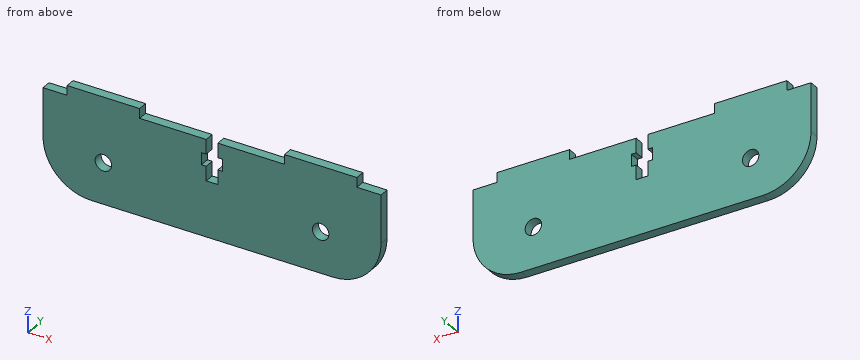
```python
from build123d import *

# Parameters (mm, degrees)
SKETCH_1_W          = 70
SKETCH_1_H          = 20
SKETCH_1_R          = 1.7
EXTRUDE_1_DEPTH     = 2
CUT_EXTRUDE_1_DEPTH = 2
SKETCH_3_W          = 15
SKETCH_3_H          = 2
EXTRUDE_2_DEPTH     = 2
FILLET_1_R          = 10


with BuildPart() as part:
    # 草图1 → 凸台-拉伸1 (new body)
    with BuildSketch(Plane(origin=(0, 0, 0), x_dir=(1, 0, 0), z_dir=(0, 1, 0))):
        with Locations((35, -10)):
            Rectangle(SKETCH_1_W, SKETCH_1_H)
        with Locations(Location((57.5, -8.5, 0), (0, 0, 270))):
            Circle(SKETCH_1_R, mode=Mode.SUBTRACT)
        with Locations(Location((12.5, -8.5, 0), (0, 0, 270))):
            Circle(SKETCH_1_R, mode=Mode.SUBTRACT)
    extrude(amount=EXTRUDE_1_DEPTH)

    # 草图2 → 切除-拉伸1 (cut)
    with BuildSketch(Plane(origin=(0, 2, 0), x_dir=(1, 0, 0), z_dir=(0, 1, 0))):
        Polygon((33.8, -20), (33.8, -17), (32.8, -17), (32.8, -14.5), (33.8, -14.5), (33.8, -11.5), (36.2, -11.5), (36.2, -14.5), (37.2, -14.5), (37.2, -17), (36.2, -17), (36.2, -20), align=None)
    extrude(amount=-CUT_EXTRUDE_1_DEPTH, mode=Mode.SUBTRACT)

    # 草图3 → 凸台-拉伸2 (add)
    with BuildSketch(Plane(origin=(0, 2, 0), x_dir=(1, 0, 0), z_dir=(0, 1, 0))):
        with Locations((12.5, -21)):
            Rectangle(SKETCH_3_W, SKETCH_3_H)
        with Locations((57.5, -21)):
            Rectangle(SKETCH_3_W, SKETCH_3_H)
    extrude(amount=-EXTRUDE_2_DEPTH)

    # 圆角1
    fillet_1_edges = [part.edges().sort_by_distance(p)[0] for p in [
        (0, 1, 0),
        (70, 1, 0),
    ]]
    fillet(fillet_1_edges, radius=FILLET_1_R)


solid = part.part
```
Geometry: final body of the model. Coordinates: model frame, mm. Give positions to 0.01 mm unless a question says otherwise; leave off trailing zeros. Loops run counter-clockwise (first coordinate to the right, second up) from the corner with the lowest first, then second, coordinate; pieces in that order, holes last. Notation, with made-up numbers: (86.25, 65.5) -> (104.25, 65.5) arc R11 ccw to (104.25, 69.5) -> close; hole circle Ø6 at (74.5, 2.5). An arc over 180 degrees is marked (long way). Return JSON: item names as keys, results as strings.
Item 1: Section B-B, the plane z = 15.5. Output: boundary loops of the cut face in (x, y), plus the area to 3 significant figures.
Filled in:
{"outline": "(0, 0) -> (32.8, 0) -> (32.8, 2) -> (0, 2) -> close; (37.2, 0) -> (70, 0) -> (70, 2) -> (37.2, 2) -> close", "area": "131 mm^2"}
Item 2: Line query: line 1 (X direction, y = 0.1, z = 13); line 2 (X direction, y = 0.4, z = 8.5); line 3 (X direction, y = 1.7, z = 20.75). Output: solid intervals per line, ascending.
Filled in:
{"line 1": "0 to 33.8, 36.2 to 70", "line 2": "0.11 to 10.8, 14.2 to 55.8, 59.2 to 69.89", "line 3": "5 to 20, 50 to 65"}
Item 3: Pin query (flat end, axial travel): P1, Ø8, axis at x = 17.5, z = 5, coming from the -Y side; P2, Ø1, axis at y = 1, z = 21.5, coming from the -X side; P3, Ø1, axis at y = 1.5, z = 21, coming from the +X side. Return the tip coordinate at first contact, or that it passes through.
Filled in:
{"P1": "y = 0", "P2": "x = 5", "P3": "x = 65"}
Item 4: Section C-C, the plane y = 0.8. Output: boundary loops of the cut face in (x, z), plus the area to 3 significant figures.
Filled in:
{"outline": "(0, 10) arc R10 ccw to (10, 0) -> (60, 0) arc R10 ccw to (70, 10) -> (70, 20) -> (65, 20) -> (65, 22) -> (50, 22) -> (50, 20) -> (36.2, 20) -> (36.2, 17) -> (37.2, 17) -> (37.2, 14.5) -> (36.2, 14.5) -> (36.2, 11.5) -> (33.8, 11.5) -> (33.8, 14.5) -> (32.8, 14.5) -> (32.8, 17) -> (33.8, 17) -> (33.8, 20) -> (20, 20) -> (20, 22) -> (5, 22) -> (5, 20) -> (0, 20) -> close; hole circle Ø3.4 at (12.5, 8.5); hole circle Ø3.4 at (57.5, 8.5)", "area": "1,370 mm^2"}
Item 5: Section A-A, the plane x = 12.5. Output: boundary loops of the cut face in (y, z).
Filled in:
{"outline": "(0, 0) -> (2, 0) -> (2, 6.8) -> (0, 6.8) -> close; (0, 10.2) -> (2, 10.2) -> (2, 22) -> (0, 22) -> close"}
Item 6: Section D-D, the plane z = 8.25. Output: boundary loops of the cut face in (x, y).
Filled in:
{"outline": "(0.15, 0) -> (10.82, 0) -> (10.82, 2) -> (0.15, 2) -> close; (14.18, 0) -> (55.82, 0) -> (55.82, 2) -> (14.18, 2) -> close; (59.18, 0) -> (69.85, 0) -> (69.85, 2) -> (59.18, 2) -> close"}
